Read the model definition and answer for the solid it produces. Units are mm, in the model's axes. Coordinates: 2 decimals unless noted, no trailing zeros. Write each loop counter-clockwise with the first axis right and the second up, starting at its lowest first coordinate (ties: lowest second). Pieces come first, ordered by that corner, then holes. Notation, with made-up numbers: (25.5, -37.75) -> (35.5, -37.75) arc R23 ccw to (35.5, -2.75) -> close; hole circle Ø9 at (-27, 17). An arc over 180 degrees is marked (long way). Answer as a JSON object with one key per item and string values. Group by question number.
(1) Flat-ended cylindrical pins translate along their axes: P1, Ø2, axis at x = 11, y = -1, coming from the -Z side; P2, Ø1.5, axis at y = -3.5, z = -8, coming from the +X side; P3, Ø1, axis at y = -2.5, z = 5.5, coming from the +X side; P4, Ø1, axis at x = -0.5, z = 7.5, coming from the +Y side. Find the tip coordinate at first contact, or state that the pin passes through.
(2) Find section A-A (z = 0). Give the vertices of the cut face in (x, y).
(3) For a pull along X with two mould halves and no side action, classify faces 1 (the face through (0, 0, -3)), 2 (the face through (2.386, -5.989, -3.987)), 3 (the face through (-4.995, -3, 0)) as +X half, -X half, draft (parallel to the pull), parting line (faces both ways), or undercut.
(4) Straight lines are drawn through the part: L1, parallel to X at y = -1.5, z = -2; L2, parallel to X at y = -2.25, z = -1.75; L3, parallel to X at y = -1.25, z = 2.5. For each, find the intervals that lie inside material, in ascending order.
(5) Find section D-D (z = -9.5). Give the vertices of the cut face in (x, y), then the cut area to 3 significant figures.
(6) Find section B-B (y = -2.5). Give the vertices of the cut face in (x, z) (1 decimal), then the cut area to 3 significant figures.
(7) Find section C-C (x = 7.25). Give the vertices of the cut face in (y, z).
from build123d import *

# Parameters (mm, degrees)
F0_R     = 3.78575
F2_DEPTH = 6.35
F3_R     = 1.341607
F4_R     = 1.20213
F5_D     = 4.445


with BuildPart() as f2:
    # F0 (on Front) + F1 (on Front) → F2 (new body)
    with BuildSketch(Plane.XZ):
        with Locations((9.935658, 0)):
            Circle(F0_R)
        with Locations((-4.967829, 8.604533)):
            Circle(F0_R)
        with Locations((-4.967829, -8.604533)):
            Circle(F0_R)
    with BuildSketch(Plane.XZ):
        Polygon((9.958743, 0), (-4.995326, 8.571174), (-4.995326, -8.656174), align=None)
    extrude(amount=F2_DEPTH)

    # F3
    f3_edges = [f2.edges().sort_by_distance(p)[0] for p in [
        (2.476077, 0, 4.288815),
        (-4.995326, 0, 0),
        (2.494509, 0, -4.320677),
    ]]
    fillet(f3_edges, radius=F3_R)

    # F4
    f4_edges = [f2.edges().sort_by_distance(p)[0] for p in [
        (-4.995326, -6.35, 0),
        (2.476077, -6.35, 4.288815),
        (2.494509, -6.35, -4.320677),
    ]]
    fillet(f4_edges, radius=F4_R)

    # F5 (through all)
    with Locations(Plane(origin=(0, 0, 0), x_dir=(1, 0, 0), z_dir=(0, 1, 0))):
        with Locations((0, 0)):
            Hole(F5_D / 2)


solid = f2.part
Results below:
{
 "1": {"P1": "stops at z = -3.79", "P2": "stops at x = -1.18", "P3": "stops at x = 1.24", "P4": "passes through"},
 "2": {"outline": "(-5, -5.15) arc R1.2 ccw to (-3.79, -6.35) -> (-2.22, -6.35) -> (-2.22, 0) -> (-3.65, 0) arc R1.34 ccw to (-5, -1.34) -> close; (2.22, -6.35) -> (13.72, -6.35) -> (13.72, 0) -> (2.22, 0) -> close"},
 "3": {"face 1": "draft", "face 2": "undercut", "face 3": "-X half"},
 "4": {"L1": "x = -5 to -0.97, 0.97 to 6.5, 6.72 to 13.15", "L2": "x = -5 to -1.37, 1.37 to 13.29", "L3": "x = -4.99 to 5.59, 7.09 to 12.78"},
 "5": {"outline": "(-8.65, -6.35) -> (-1.29, -6.35) -> (-1.29, 0) -> (-8.65, 0) -> close", "area": "46.7 mm2"},
 "6": {"outline": "(-5, -4.8) arc R3.8 ccw (long way) to (-1.7, -6.7) -> (6.7, -1.9) arc R3.8 ccw (long way) to (6.7, 1.9) -> (-1.7, 6.7) arc R3.8 ccw (long way) to (-5, 4.8) -> close; hole circle Ø4.4 at (0, 0)", "area": "226 mm2"},
 "7": {"outline": "(-6.35, -2.67) -> (0, -2.67) -> (0, 2.67) -> (-6.35, 2.67) -> close"}
}
